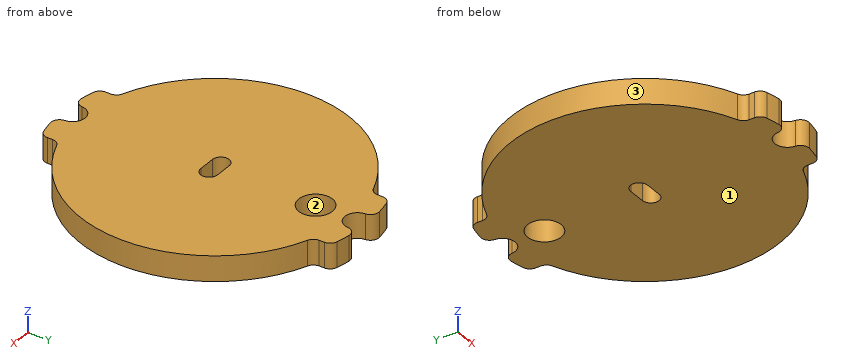
Autodesk Inventor part; units mm, degrees
ref_plane "YZ Plane" through (0, 0, 0) normal (1, 0, 0) x (0, 1, 0)
ref_plane "XZ Plane" through (0, 0, 0) normal (0, 1, 0) x (-1, 0, 0)
ref_plane "XY Plane" through (0, 0, 0) normal (0, 0, 1) x (1, 0, 0)
sketch "Sketch1" plane through (0, 0, 0) normal (0, 0, 1) x (1, 0, 0)
  circle A0 centre (0, 12) radius 2
  arc A1 (-5.6471, 14.9703) -> (-5.6471, -14.9703) centre (0, 0) ccw
  arc A2 (5.6471, -14.9703) -> (5.6471, 14.9703) centre (0, 0) ccw
  line L0 (-5, -16.5227) -> (-5, -15.906)
  line L1 (-5, 15.906) -> (-5, 16.5227)
  line L2 (5, 16.5227) -> (5, 15.906)
  line L3 (5, -15.906) -> (5, -16.5227)
  arc A3 (-5.6471, 14.9703) -> (-5, 15.906) centre (-6, 15.906) ccw
  arc A4 (-4.2353, 17.4946) -> (-5, 16.5227) centre (-4, 16.5227) ccw
  arc A5 (5, 16.5227) -> (4.2353, 17.4946) centre (4, 16.5227) ccw
  arc A6 (5, 15.906) -> (5.6471, 14.9703) centre (6, 15.906) ccw
  arc A7 (5.6471, -14.9703) -> (5, -15.906) centre (6, -15.906) ccw
  arc A8 (4.2353, -17.4946) -> (5, -16.5227) centre (4, -16.5227) ccw
  arc A9 (-5, -16.5227) -> (-4.2353, -17.4946) centre (-4, -16.5227) ccw
  arc A10 (-5, -15.906) -> (-5.6471, -14.9703) centre (-6, -15.906) ccw
  arc A11 (-1.4959, 16.8897) -> (1.4959, 16.8897) centre (0, 17) ccw
  arc A12 (1.4959, -16.8897) -> (-1.4959, -16.8897) centre (0, -17) ccw
  arc A13 (4.2353, 17.4946) -> (2.6399, 17.8054) centre (0, 0) ccw
  arc A14 (-2.6399, 17.8054) -> (-4.2353, 17.4946) centre (0, 0) ccw
  arc A15 (-4.2353, -17.4946) -> (-2.6399, -17.8054) centre (0, 0) ccw
  arc A16 (2.6399, -17.8054) -> (4.2353, -17.4946) centre (0, 0) ccw
  arc A17 (-2.6399, -17.8054) -> (-1.4959, -16.8897) centre (-2.4932, -16.8162) ccw
  arc A18 (1.4959, -16.8897) -> (2.6399, -17.8054) centre (2.4932, -16.8162) ccw
  arc A19 (-1.4959, 16.8897) -> (-2.6399, 17.8054) centre (-2.4932, 16.8162) ccw
  arc A20 (2.6399, 17.8054) -> (1.4959, 16.8897) centre (2.4932, 16.8162) ccw
  arc A21 (-1, 1) -> (-1, -1) centre (-1, 0) ccw
  arc A22 (1, -1) -> (1, 1) centre (1, 0) ccw
  line L4 (-1, 1) -> (1, 1)
  line L5 (1, -1) -> (-1, -1)
  point P0 (-5, 17.2916)
  point P1 (5, -17.2916)
  point P2 (5, 17.2916)
  point P3 (-5, -17.2916)
  point P4 (5, 15.1987)
  point P5 (-5, 15.1987)
  point P6 (-5, -15.1987)
  point P7 (5, -15.1987)
  dimension "d6" = 4
  dimension "d16" = 1
  dimension "d17" = 16
  dimension "d18" = 16
  dimension "d21" = 10
  dimension "d22" = 10
  dimension "d25" = 3
  dimension "d28" = 3
  dimension "d29" = 1
  dimension "d34" = 12
  dimension "d35" = 2
  dimension "d36" = 2
extrude "Extrusion4" add sketch "Sketch1" along normal blind 3
properties part number "Outer Endcap080513" material "Polycarbonate, Clear"
Could you check a few things on this model? Use its own coordinates, in mm. Face numbers are marked on the shaded views. Round coordinates to 2 decimals unless told otherwise and drop trailing zeros. Write each loop counter-clockwise with the first axis right and the second up, starting at its lowest first coordinate (ties: lowest second). Pieces come first, ordered by that corner, then holes. Notation, with made-up numbers: (3, 11) - (26, 11) arc R26 cw to (26, 45) - close; hole circle Ø11 at (73, 71.5). An arc over 180 degrees is marked (long way). Use a Markdown table: item, result.
Q1. I want a section at D-D (y = 12). List the corners of the cut face in (x, z) for me, plus the area to 3 significant figures.
Output values:
| item | result |
|---|---|
| outline | (-10.58, 0) - (-2, 0) - (-2, 3) - (-10.58, 3) - close; (2, 0) - (10.58, 0) - (10.58, 3) - (2, 3) - close |
| area | 51.5 mm2 |
Q2. I want a section at C-C (z = 1). Count the separate pieces of the cut face and the enclosed holes in it, plus the area to 3 significant figures.
Output values:
| item | result |
|---|---|
| separate pieces | 1 |
| enclosed holes | 2 |
| area | 811 mm2 |
Q3. For pin 1 (0.6 mm diameter, centred on x = 0, z = 1, fed in from +Y); pin 2 (6.5 mm diameter, centred on x = 0, y = 12, fed in from +Z); pin 3 (0.6 mm diameter, centred on x = 0, z = 1, fed in from -Y); pin 4 (1.5 mm diameter, centred on x = 12.5, z = 0.5, fed in from +Y), each with a flat end and sliding along its axis, tell me the tip position at first contact or that it passes through.
Output values:
| item | result |
|---|---|
| pin 1 | y = 15.53 |
| pin 2 | z = 3 |
| pin 3 | y = -15.53 |
| pin 4 | y = 10.86 |
Q4. Thinking about a two-plate mould opening in Y: for the marked faces 1, 2 and 3, which applies, released by +Y, released by -Y, zero draft, split by the parting line, or undercut?
Output values:
| item | result |
|---|---|
| face 1 | zero draft |
| face 2 | undercut |
| face 3 | split by the parting line |
Q5. I want a section at B-B (y = 0). List the corners of the cut face in (x, z) for me, plus the area to 3 significant figures.
Output values:
| item | result |
|---|---|
| outline | (-16, 0) - (-2, 0) - (-2, 3) - (-16, 3) - close; (2, 0) - (16, 0) - (16, 3) - (2, 3) - close |
| area | 84.0 mm2 |
Q6. Please list where these lines run through material, in increasing order: L1, parallel to X at y = -5, z = 1.2; L2, parallel to Y at x = 13.5, z = 1; L3, parallel to X at y = 11.5, z = 2.8.
Output values:
| item | result |
|---|---|
| L1 | -15.2 to 15.2 |
| L2 | -8.59 to 8.59 |
| L3 | -11.12 to -1.94, 1.94 to 11.12 |
Q7. I want a section at A-A (x = 0). List the corners of the cut face in (y, z) for me, plus the area to 3 significant figures.
Output values:
| item | result |
|---|---|
| outline | (-15.5, 0) - (-1, 0) - (-1, 3) - (-15.5, 3) - close; (1, 0) - (10, 0) - (10, 3) - (1, 3) - close; (14, 0) - (15.5, 0) - (15.5, 3) - (14, 3) - close |
| area | 75.0 mm2 |
